CAD build for the part. Positions are in the model's coordinates, mm. A direction names the side the tool comes from. Give positions to 0.01 mm unless a question says otherwise; leave off trailing zeros. Write each loop counter-clockwise with the first axis right and the second up, starting at its lowest first coordinate (ties: lowest second). Pieces come first, ordered by that corner, then holes. Notation, with made-up numbers: (8.5, -8) -> (53.5, -8) arc R23 ccw to (53.5, 28) -> close; hole circle Ø11 at (21.5, -8.5). An arc over 180 degrees is marked (long way). Answer in a Markdown table with one row per item. Add a question column.
```python
from build123d import *

# Parameters (mm, degrees)
F0_W     = 40
F0_H     = 40
F0_R     = 1.4732
F0_W_2   = 10.15
F0_H_2   = 1.74625
F0_W_3   = 1.74625
F0_H_3   = 10.15
F1_DEPTH = 0.79375
F2_R     = 5


# Not quite as in the source:
# - a length typed as a fraction of an inch, garbled in the dataset ("3 / 203.2 mm" for 3/8 in), is restored


with BuildPart() as f1:
    # F0 (on Right) → F1 (new body, symmetric)
    with BuildSketch(Plane.YZ):
        Rectangle(F0_W, F0_H)
        with Locations((-15, -15)):
            Circle(F0_R, mode=Mode.SUBTRACT)
        with BuildLine():
            ThreePointArc((-4.8291651246, -3.25), (-6.4019057856, -3.4570552361), (-4.9363448016, -2.85))
            ThreePointArc((-4.9363448016, -2.85), (-4.8564244636, -3.0429447639), (-4.8291651246, -3.25))
        make_face(mode=Mode.SUBTRACT)
        with Locations((0, -15)):
            Rectangle(F0_W_2, F0_H_2, mode=Mode.SUBTRACT)
        with Locations((15, -15)):
            Circle(F0_R, mode=Mode.SUBTRACT)
        with BuildLine():
            ThreePointArc((6.4291651246, -3.25), (5.4221098885, -4.022740661), (4.9363448016, -2.85))
            ThreePointArc((4.9363448016, -2.85), (5.8362203607, -2.477259339), (6.4291651246, -3.25))
        make_face(mode=Mode.SUBTRACT)
        with Locations((-15, 15)):
            Circle(F0_R, mode=Mode.SUBTRACT)
        with BuildLine():
            ThreePointArc((0, 5), (3.5355339059, 3.5355339059), (5, 0))
            ThreePointArc((5, 0), (4.8296291314, -1.2940952255), (4.3301270189, -2.5))
            ThreePointArc((4.3301270189, -2.5), (0, -5), (-4.3301270189, -2.5))
            ThreePointArc((-4.3301270189, -2.5), (-4.3301270189, 2.5), (0, 5))
        make_face(mode=Mode.SUBTRACT)
        with BuildLine():
            ThreePointArc((0.8, 6.5), (0.5656854249, 5.9343145751), (0, 5.7))
            ThreePointArc((0, 5.7), (-0.5656854249, 7.0656854249), (0.8, 6.5))
        make_face(mode=Mode.SUBTRACT)
        with Locations((15, 0)):
            Rectangle(F0_W_3, F0_H_3, mode=Mode.SUBTRACT)
        with Locations((0, 15)):
            Rectangle(F0_W_2, F0_H_2, mode=Mode.SUBTRACT)
        with Locations((15, 15)):
            Circle(F0_R, mode=Mode.SUBTRACT)
    extrude(amount=F1_DEPTH, both=True)

    # F2
    f2_edges = [f1.edges().sort_by_distance(p)[0] for p in [
        (0, -20, 20),
        (0, 20, 20),
        (0, -20, -20),
        (0, 20, -20),
    ]]
    fillet(f2_edges, radius=F2_R)


solid = f1.part
```
Item 1: Slice it at C-C, the plane y = -17. List the corners of the cut face in (x, z), then the cut area to 3 significant figures.
Item 2: Which spindle directions (+Z, -Z, +X, -X, +Y, -Y) get a long thin tool onto all of the face, cutting with end or side? Do faces 4 (the face through (0, -20, 0)), 5 (the face through (0, 14.127, 0)). Say none if no direction does.
Item 3: Drop flat-ended pins along their axis: pin 1 Ø0.5 at (x, y) = (0.5, 15.5) entering from -Z; pin 2 Ø2.5 at (y, z) = (-15, 15) entering from -X. Give the stop position or say it passes through.
Item 4: Slice it at A-A, the plane z = 6.5. List the corners of the cut face in (x, y).
Item 5: Slice it at B-B, the plane x = 0.4. State how many separate pieces and enclosed holes the cut face has, then the cut area to 3 significant figures.
Item 6: Probe L1, parallel to Z at x = -0.2, y = -15; L2, parallel to Y at x = 0.65, z = -3.25; L3, parallel to Y at x = 0.4, z = -15.5 (3 decimals). List the from-to ranges inside material, lowest first. Write a range as from..to.
Item 7: Mould opens along Z. For faces 1 (the face through (0.794, -5, -4)), 2 (the face through (0, -19, -18)), 3 (the face through (0, 0, 14.127)) say: released by +Z, released by -Z, zero draft, split by the parting line, or undercut.
Answer key:
| question | item | result |
|---|---|---|
| 1 | outline | (-0.79, -19.58) -> (0.79, -19.58) -> (0.79, 19.58) -> (-0.79, 19.58) -> close |
| 1 | area | 62.2 mm² |
| 2 | face 4 | +Z, -Z, +X, -X, -Y |
| 2 | face 5 | +X, -X |
| 3 | pin 1 | stops at z = -19.99 |
| 3 | pin 2 | passes through |
| 4 | outline | (-0.79, -20) -> (0.79, -20) -> (0.79, -0.8) -> (-0.79, -0.8) -> close; (-0.79, 0.8) -> (0.79, 0.8) -> (0.79, 20) -> (-0.79, 20) -> close |
| 5 | separate pieces | 1 |
| 5 | enclosed holes | 11 |
| 5 | area | 1,410 mm² |
| 6 | L1 | z = -20..-16.47, -13.53..13.53, 16.47..20 |
| 6 | L2 | y = -20..-6.43, -4.83..-3.8, 3.8..4.83, 6.43..14.13, 15.87..20 |
| 6 | L3 | y = -19.975..-16.386, -13.614..-5.075, 5.075..13.614, 16.386..19.975 |
| 7 | face 1 | zero draft |
| 7 | face 2 | released by -Z |
| 7 | face 3 | undercut |
